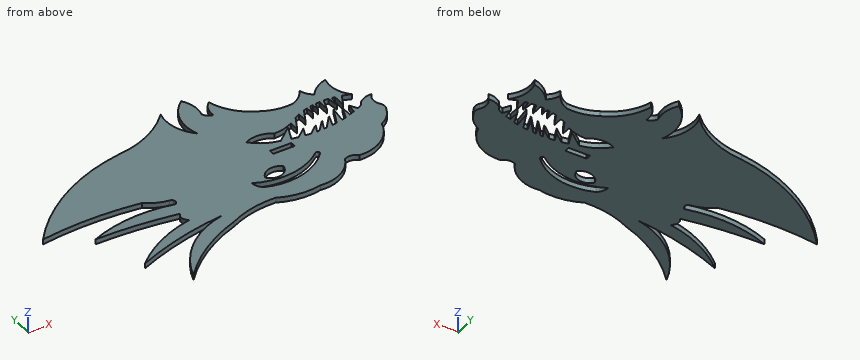
```python
from build123d import *

# Parameters (mm, degrees)
SKETCH1_W           = 6.35
SKETCH1_H           = 1.524
BOSS_EXTRUDE1_DEPTH = 1.524


with BuildPart() as part:
    # Sketch1 → Boss-Extrude1 (new body)
    with BuildSketch(Plane.XY):
        with BuildLine():
            Line((-118.967464928, 3.837147512), (-120.210313768, 5.894153968))
            Line((-120.210313768, 5.894153968), (-120.507329985, 3.167212811))
            Line((-120.507329985, 3.167212811), (-122.125463269, 2.558958735))
            Line((-122.125463269, 2.558958735), (-122.125463269, 5.894153968))
            Line((-122.125463269, 5.894153968), (-123.701040917, 1.954785522))
            Line((-123.701040917, 1.954785522), (-124.938272303, 1.633539151))
            Line((-124.938272303, 1.633539151), (-124.405721371, 6.522952497))
            Line((-124.405721371, 6.522952497), (-126.85553137, 1.234027863))
            Line((-126.85553137, 1.234027863), (-128.185864984, 1.075304442))
            Line((-128.185864984, 1.075304442), (-126.85553137, 4.86565074))
            Line((-126.85553137, 4.86565074), (-130.098565327, 0.850073658))
            Line((-130.098565327, 0.850073658), (-130.926497191, 0.78728846))
            Line((-130.926497191, 0.78728846), (-129.340887254, 4.210481059))
            Line((-129.340887254, 4.210481059), (-132.319280434, 0.722942299))
            Line((-132.319280434, 0.722942299), (-133.020376887, 0.72112245))
            Line((-133.020376887, 0.72112245), (-131.834849185, 3.28057264))
            Line((-131.834849185, 3.28057264), (-134.796306141, 0.76870718))
            Line((-134.796306141, 0.76870718), (-136.410777473, 0.933118092))
            Line((-136.410777473, 0.933118092), (-135.265463132, 3.678674725))
            Line((-135.265463132, 3.678674725), (-138.261220774, 1.137715912))
            Line((-138.261220774, 1.137715912), (-140.197350719, 1.50653427))
            Line((-140.197350719, 1.50653427), (-138.261220774, 6.147840352))
            Line((-138.261220774, 6.147840352), (-142.88987797, 2.221879477))
            ThreePointArc((-142.88987797, 2.221879477), (-147.08283508, 3.64953129), (-150.612134583, 6.325932612))
            ThreePointArc((-150.612134583, 6.325932612), (-146.485856937, 7.203077476), (-142.522861876, 5.757317996))
            ThreePointArc((-142.522861876, 5.757317996), (-139.511076326, 6.147840352), (-136.689748679, 7.271882262))
            Line((-136.689748679, 7.271882262), (-136.689748679, 4.31406956))
            Line((-136.689748679, 4.31406956), (-134.379090787, 8.749235121))
            ThreePointArc((-134.379090787, 8.749235121), (-133.626205107, 9.140656329), (-132.857462763, 9.499937023))
            Line((-132.857462763, 9.499937023), (-132.857462763, 6.530588828))
            Line((-132.857462763, 6.530588828), (-130.926497191, 10.236958357))
            ThreePointArc((-130.926497191, 10.236958357), (-130.345173873, 10.415525196), (-129.75871249, 10.576416347))
            Line((-129.75871249, 10.576416347), (-129.75871249, 7.796759722))
            Line((-129.75871249, 7.796759722), (-128.644783844, 10.830408865))
            ThreePointArc((-128.644783844, 10.830408865), (-128.214678718, 10.910834307), (-127.782924128, 10.981874047))
            Line((-127.782924128, 10.981874047), (-127.782924128, 8.576451057))
            Line((-127.782924128, 8.576451057), (-126.85553137, 11.102092407))
            ThreePointArc((-126.85553137, 11.102092407), (-126.258208322, 11.156424297), (-125.659529634, 11.192901774))
            Line((-125.659529634, 11.192901774), (-125.659529634, 7.796759722))
            Line((-125.659529634, 7.796759722), (-124.405721372, 11.211353983))
            ThreePointArc((-124.405721372, 11.211353983), (-123.721315902, 11.188391312), (-123.038090537, 11.142117871))
            Line((-123.038090537, 11.142117871), (-122.625154661, 7.796759722))
            Line((-122.625154661, 7.796759722), (-122.125463269, 11.04361803))
            ThreePointArc((-122.125463269, 11.04361803), (-121.68108693, 10.980301708), (-121.238235987, 10.907073779))
            Line((-121.238235987, 10.907073779), (-121.238235987, 7.074194908))
            Line((-121.238235987, 7.074194908), (-119.450305834, 10.506016758))
            ThreePointArc((-119.450305834, 10.506016758), (-118.170254613, 10.11057495), (-116.919404117, 9.630701645))
            ThreePointArc((-116.919404117, 9.630701645), (-119.349830951, 13.774572734), (-119.242407582, 18.577395072))
            ThreePointArc((-119.242407582, 18.577395072), (-122.479801343, 17.135418403), (-125.032625503, 14.677145863))
            ThreePointArc((-125.032625503, 14.677145863), (-126.511437413, 16.117497101), (-127.319227749, 18.017226326))
            ThreePointArc((-127.319227749, 18.017226326), (-129.072821157, 15.778913608), (-131.451278595, 14.220685806))
            ThreePointArc((-131.451278595, 14.220685806), (-136.013842114, 14.266990808), (-140.318864701, 15.778913608))
            Line((-140.318864701, 15.778913608), (-140.572063038, 15.900311384))
            ThreePointArc((-140.572063038, 15.900311384), (-146.082089593, 19.986277928), (-149.28772088, 26.05088371))
            ThreePointArc((-149.28772088, 26.05088371), (-150.98225883, 23.655808523), (-151.240302387, 20.733265531))
            ThreePointArc((-151.240302387, 20.733265531), (-152.718101686, 21.336819353), (-153.601407922, 22.66645768))
            ThreePointArc((-153.601407922, 22.66645768), (-153.396919216, 26.552679329), (-154.91417797, 30.136317175))
            ThreePointArc((-154.91417797, 30.136317175), (-159.291131596, 23.805118938), (-158.91395171, 16.117497101))
            ThreePointArc((-158.91395171, 16.117497101), (-162.327187611, 21.593822413), (-162.381546066, 28.046524436))
            ThreePointArc((-162.381546066, 28.046524436), (-170.625215942, 21.84762456), (-180.560631507, 19.077792393))
            ThreePointArc((-180.560631507, 19.077792393), (-200.503081439, 12.098235462), (-216.39853294, -1.821180682))
            ThreePointArc((-216.39853294, -1.821180682), (-201.656488756, -0.752866976), (-186.914444571, -1.821180682))
            ThreePointArc((-186.914444571, -1.821180682), (-183.850945452, -3.661612396), (-180.414923023, -4.644447892))
            ThreePointArc((-180.414923023, -4.644447892), (-179.359692742, -5.560033265), (-180.052236488, -6.773371915))
            ThreePointArc((-180.052236488, -6.773371915), (-192.817706831, -5.844622664), (-205.252520527, -8.876984225))
            ThreePointArc((-205.252520527, -8.876984225), (-193.210647633, -9.328958481), (-181.263188413, -10.900327847))
            ThreePointArc((-181.263188413, -10.900327847), (-181.878443359, -12.812123131), (-180.664874061, -14.412357306))
            ThreePointArc((-180.664874061, -14.412357306), (-191.17895358, -17.957183031), (-200.243848586, -24.35556846))
            ThreePointArc((-200.243848586, -24.35556846), (-186.726305796, -19.732822879), (-172.667325525, -17.19534115))
            ThreePointArc((-172.667325525, -17.19534115), (-185.150029357, -23.504388145), (-192.700842194, -35.277543815))
            ThreePointArc((-192.700842194, -35.277543815), (-183.0911903, -26.748605396), (-171.570271252, -21.060317047))
            ThreePointArc((-171.570271252, -21.060317047), (-164.623433194, -18.575118247), (-157.275939172, -17.904966269))
            ThreePointArc((-157.275939172, -17.904966269), (-151.145420538, -19.702741956), (-144.764510502, -19.387712987))
            ThreePointArc((-144.764510502, -19.387712987), (-138.075773009, -18.065674232), (-133.430936261, -13.074433174))
            ThreePointArc((-133.430936261, -13.074433174), (-131.329864526, -12.686756633), (-129.424108432, -13.652618554))
            ThreePointArc((-129.424108432, -13.652618554), (-121.886353154, -11.514694937), (-117.426632435, -5.072695004))
            ThreePointArc((-117.426632435, -5.072695004), (-114.82444132, -3.21357396), (-113.136821812, -0.497019148))
            ThreePointArc((-113.136821812, -0.497019148), (-112.701188688, 0.934666439), (-113.136821812, 2.366352026))
            ThreePointArc((-113.136821812, 2.366352026), (-113.78472542, 4.800381574), (-112.701188688, 7.074194908))
            ThreePointArc((-112.701188688, 7.074194908), (-114.988500666, 6.766664074), (-116.919404117, 5.502550489))
            ThreePointArc((-116.919404117, 5.502550489), (-117.728663328, 4.405730062), (-118.967464928, 3.837147512))
        make_face()
        with Locations((-144.335438151, -0.762)):
            Rectangle(SKETCH1_W, SKETCH1_H, mode=Mode.SUBTRACT)
        with BuildLine():
            ThreePointArc((-137.559244953, -7.819206053), (-146.689526794, -13.235024078), (-157.275939172, -12.446985783))
            ThreePointArc((-157.275939172, -12.446985783), (-158.429212855, -11.102896957), (-158.91395171, -9.399475928))
            ThreePointArc((-158.91395171, -9.399475928), (-148.192505964, -11.193493039), (-138.261220774, -6.773371915))
            ThreePointArc((-138.261220774, -6.773371915), (-137.447536507, -6.985721903), (-137.559244953, -7.819206053))
        make_face(mode=Mode.SUBTRACT)
        with BuildLine():
            ThreePointArc((-148.216931549, -7.339340233), (-151.974990586, -6.526199766), (-154.789067747, -9.14634764))
            ThreePointArc((-154.789067747, -9.14634764), (-150.886892893, -10.483641343), (-148.216931549, -7.339340233))
        make_face(mode=Mode.SUBTRACT)
    extrude(amount=BOSS_EXTRUDE1_DEPTH)


solid = part.part
```
Check sheet for the modelled part. Datum: model origin and axes. Units: mm. Round coordinates to 2 decimals unless told otherwise and drop trailing zeros. Order: outer loops, then holes, each group sorted by start corner. A loop starts at its lowest first (then second) coordinate and runs counter-clockwise, first axis right, second up. Notation, with made-up numbers: (2.25, 89.25) - (40.25, 89.25) arc R18 ccw to (40.25, 106.25) - close; hole circle Ø9 at (58.5, 34.25). An arc over 180 degrees is marked (long way). Write item = value, one per line.
Q1. Go/stop test with flat-tipped pins: pin 1 (0.5 mm diameter, centred on y = 9.5, z = 0.5, fed in from -X); pin 2 (0.5 mm diameter, centred on y = 5, z = 1, fed in from +X); pin 3 (0.8 mm diameter, centred on y = 9.5, z = 1, fed in from -X). Record where each tip stops, or that it passes through.
Computed:
pin_1 = -204.9
pin_2 = -113.71
pin_3 = -205.11
Q2. Section check B-B (y = -16). Record the boundary of the cut face in (x, z), and give its area (3 significant figures).
Computed:
outline = (-186.62, 0) - (-135.42, 0) - (-135.42, 1.52) - (-186.62, 1.52) - close
area = 78.0 mm^2
Q3. Thickness scan on line 1 along Y through (x, z) = (-152.5, 0.8); line 2 along X through (y, z) = (23, 0.65); line 3 along Y through (x, z) = (-196.5, 0.5). Record the ranges inside material, lowest first.
Computed:
line_1 = -19.49 to -13.61, -11.25 to -10.56, -6.71 to 21.18
line_2 = -168.52 to -162.65, -159.49 to -153.51, -151.18 to -148.11
line_3 = -22.84 to -21.23, -9.09 to -6.32, -0.88 to 14.22
Q4. Section check A-A (z = 0.7). State how many separate pieces and enclosed holes the cut face has, and give its area (3 significant figures).
Computed:
separate_pieces = 1
enclosed_holes = 3
area = 2,790 mm^2
